Autodesk Inventor part; units mm, degrees
ref_plane "Work Plane1" through (-381, 0, 274.6375) normal (0, 0, 1) x (1, 0, 0)
ref_plane "YZ Plane" through (0, 0, 0) normal (1, 0, 0) x (0, 1, 0)
ref_plane "XZ Plane" through (0, 0, 0) normal (0, 1, 0) x (-1, 0, 0)
sketch "Sketch1" plane through (0, 0, 0) normal (0, 1, 0) x (-1, 0, 0)
  line L0 (-381, 304.8) -> (-381, -304.8)
  line L1 (-381, -304.8) -> (381, -304.8)
  line L2 (381, -304.8) -> (381, 304.8)
  line L3 (381, 304.8) -> (-381, 304.8)
  line L4 (-381, 304.8) -> (381, -304.8) construction
  line L5 (-381, -304.8) -> (381, 304.8) construction
  point P0 (0, 0)
  dimension "width" = 609.6
  dimension "length" = 762
extrude "Extrusion1" add sketch "Sketch1" against normal blind 6.35
ref_plane "Work Plane1" through (-381, 0, 274.6375) normal (0, 0, 1) x (1, 0, 0)
sketch "Sketch2" plane through (0, 0, 0) normal (0, 1, 0) x (1, 0, 0)
  line L0 (-254.5026, 247.65) -> (138.8237, 247.65)
  line L1 (284.8737, 101.6) -> (284.8737, -279.4)
  arc A0 (284.8737, 101.6) -> (138.8237, 247.65) centre (138.8237, 101.6) ccw
  line L2 (-381, -304.8) -> (381, -304.8)
  point P0 (0, 0)
  dimension "d4" = 292.1
  dimension "d5" = 381
  dimension "d6" = 558.8
  dimension "d10" = 25.4
sketch "Sketch3" plane through (-381, 0, 274.6375) normal (0, 0, 1) x (1, 0, 0)
  line L0 (665.6905, 0) -> (699.5621, 0)
  line L1 (699.5621, 0) -> (699.5621, 50.8385)
  line L2 (699.5621, 50.8385) -> (665.6905, 50.8385)
  line L3 (665.6905, 50.8385) -> (665.6905, 0)
  point P0 (381, 0)
sweep "Sweep1" add profiles "Sketch3" path "Sketch2" path curves L1 A0 L0
properties part number "ShooterBase" material "Wood (Birch)"
Source: CAD feature listing. Evaluate the final solid. Frame: model axes, mm. A direction names the side the tool comes from. Give positions to 0.01 mm unless a question says otherwise; leave off trailing zeros. Write each loop counter-clockwise with the first axis right and the second up, starting at its lowest first coordinate (ties: lowest second). Pieces come first, ordered by that corner, then holes. Notation, with made-up numbers: (4.25, 28) - (54.25, 28) arc R21 ccw to (54.25, 53) - close; hole circle Ø2 at (-38.5, 22). An arc over 180 degrees is marked (long way). One line per item, written item: value. Start each with the question number.
Q1. Set-up query: faces 4 (the face through (-254.503, 25, -265)), 5 (the face through (240.8, 25.1, -205.9)), 6 (the face through (318.562, 25, 92)). Return all of +Z, -Z, +X, -X, +Y, -Y with unobstructed straight access to the full face (end or side cutting, diameter ignored); none if empty.
Q2. Section query B-B, the plane z = -75. Return the cut outline in (x, y), then the cut area to 3 significant figures.
Q3. Draft query along Y for faces 1 (the face through (-55, 26, -247.467)), 2 (the face through (139, 50.838, -251)), 3 (the face through (5, -6.35, 4)). Return one class per face: +Y half, -Y half, draft (parallel to the pull), parting line (faces both ways), or undercut.
Q4. Section query C-C, the plane x = -270. Return the cut outline in (y, z).
Q5. First-contact query: pin 1 Ø4 at (x, z) = (-66.5, 198) entering from +Y; pin 2 Ø4 at (x, y) = (271.5, 39.5) entering from -Z; pin 3 Ø17 at (x, y) = (301.5, 27) entering from +Z. Flat tips, straight axial feed; report the tip coordinate or a pass-through.
Q6. Material intervals for probe 1 along Y at (x, z) = (-177, -79.5); probe 2 along Z at (x, y) = (-129.5, 20.5); probe 3 along X at (y, z) = (5, -108.5), sorted ascending. Write a range as from..to.
Q7. Section query A-A, the plane y = 42. Return the cut outline in (x, z).
Answer:
1. face 4: +Z, -Z, -X, +Y
1. face 5: +Z, -X, +Y
1. face 6: +Z, -Z, +X, +Y
2. outline: (-381, -6.35) - (381, -6.35) - (381, 0) - (318.56, 0) - (318.56, 50.84) - (284.69, 50.84) - (284.69, 0) - (-381, 0) - close
2. area: 6,560 mm2
3. face 1: draft
3. face 2: +Y half
3. face 3: -Y half
4. outline: (-6.35, -304.8) - (0, -304.8) - (0, 304.8) - (-6.35, 304.8) - close
5. pin 1: stops at y = 0
5. pin 2: stops at z = -225.01
5. pin 3: stops at z = 279.4
6. probe 1: y = -6.35..0
6. probe 2: z = -281.34..-247.47
6. probe 3: x = 284.53..318.43
7. outline: (-254.5, -281.34) - (138.82, -281.34) arc R179.74 ccw to (318.56, -101.6) - (318.56, 279.4) - (284.69, 279.4) - (284.69, -101.6) arc R145.87 cw to (138.82, -247.47) - (-254.5, -247.47) - close
